Could you check a few things on this model? Use its own coordinates, in mm. A direction names the side the tool comes from. Round coordinates to 2 decimals unless told otherwise and drop trailing zeros. Write each loop counter-clockwise with the first axis right and the second up, starting at its lowest first coordinate (ties: lowest second). Pieces come first, ordered by that corner, then holes. Notation, with made-up numbers: (80.25, 78) -> (96.25, 78) arc R11 ccw to (96.25, 92) -> close; hole circle Ø2 at (23, -13). An arc over 180 degrees is marked (long way). Answer as CSV lines item,"result". Start each with the question number.
Q1. Imagine slicing it at D-D on z = 0.75. Please give me the cut outline in (x, y), and give its area (3 significant figures).
Q2. For faces 1 (the flat face through (11, 2, -2)), 2 (the flat face through (2, 11, -2)), 3 (the conical face through (4.62, -11.04, -2.03)), 4 (the flat face through (8, 8, 0)), which set-ups out of +Z, -Z, +X, -X, +Y, -Y let a thin tool reach every point of the face, with its end or its side?
Q3. Imagine slicing it at A-A on x = 0. Please give me the cut outline in (y, z), and give its area (4 significant figures).
Q4. Will these pins go through, and if not, where does the flat tip stop? pin 1 Ø1 at (y, z) = (-2, -1.5) entering from -X; pin 2 Ø3 at (x, z) = (-4, 0) entering from -Y (3 decimals); pin 3 Ø5 at (x, y) = (1, -6.5) entering from +Z; pin 4 Ø2 at (x, z) = (-9.5, 1.5) entering from -Y.
Q5. If I drill on line 1 (Y direction, x = 0, z = 1.75); line 2 (Y direction, x = -11, z = -1.25); line 3 (X direction, y = 3.25, z = -2.25), over which ranges is the centre line in solid material (lowest first)? Write a range as [from, to].
Q6. Imagine slicing it at C-C on z = -3.25. Give the number of separate pieces and of enclosed holes in the cut face, and give its area (3 significant figures).
from build123d import *

# Parameters (mm, degrees)
F0_R            = 14
F0_R_2          = 10
F1_DEPTH        = 4
F2_R            = 14
F2_R_2          = 10
F3_DEPTH        = 4
F4_SIZE         = 0.5
F5_SIZE         = 3.99999
F6_W            = 4
F6_H            = 40
F7_DEPTH        = 4.001
F7_COPIES_COUNT = 4
F7_COPIES_ANGLE = 135


# Not quite as in the source:
# - a fillet or chamfer is up to 0.001 mm smaller than in the source, because OpenCascade refuses the exact size
# - a pattern or mirror of a feature is missing from the dataset's text; its kind, count and spacing are read off the source's solid


with BuildPart() as f1:
    # F0 (on Top) → F1 (new body)
    with BuildSketch(Plane.XY):
        Circle(F0_R)
        Circle(F0_R_2, mode=Mode.SUBTRACT)
    extrude(amount=F1_DEPTH)

    # F2 (on face) → F3 (join)
    with BuildSketch(Plane(origin=(0, 0, 0), x_dir=(1, 0, 0), z_dir=(0, 0, -1))):
        Circle(F2_R)
        Circle(F2_R_2, mode=Mode.SUBTRACT)
    extrude(amount=F3_DEPTH)

    # F4
    f4_edges = [f1.edges().sort_by_distance(p)[0] for p in [
        (-10, 0, 4),
    ]]
    chamfer(f4_edges, length=F4_SIZE)

    # F5 (size 4 in the source; OpenCascade refuses exactly that, so slightly less here)
    f5_edges = [f1.edges().sort_by_distance(p)[0] for p in [
        (-14, 0, -4),
    ]]
    chamfer(f5_edges, length=F5_SIZE)

    # F6 (on Top) → F7 (cut, through all)
    with BuildSketch(Plane.XY):
        Rectangle(F6_W, F6_H)
    f7 = extrude(amount=-F7_DEPTH, mode=Mode.SUBTRACT)

    # F7_copies: F7 ×4 about axis
    f7_copies_axis = Axis((0, 0, 0), (0, 0, 1))
    for i in range(1, F7_COPIES_COUNT):
        add(f7.rotate(f7_copies_axis, i * F7_COPIES_ANGLE / (F7_COPIES_COUNT - 1)), mode=Mode.SUBTRACT)


solid = f1.part
Checks:
1,outline,"circle Ø28 at (0, 0); hole circle Ø20 at (0, 0)"
1,area,"302 mm^2"
2,face 1,"-Z, +X, -X"
2,face 2,"-Z, +Y, -Y"
2,face 3,"-Z, +X, -Y"
2,face 4,"-Z"
3,outline,"(-14, 0) -> (-10, 0) -> (-10, 3.5) -> (-10.5, 4) -> (-14, 4) -> close; (10, 0) -> (14, 0) -> (14, 4) -> (10.5, 4) -> (10, 3.5) -> close"
3,area,"31.75 mm^2"
4,pin 1,"x = -12.85"
4,pin 2,"y = -13.775"
4,pin 3,"through"
4,pin 4,"y = -11.12"
5,line 1,"[-14, -10], [10, 14]"
5,line 2,"[-6.45, -2], [2, 6.45]"
5,line 3,"[-11.29, -9.46], [9.46, 11.29]"
6,separate pieces,"8"
6,enclosed holes,"0"
6,area,"24.7 mm^2"
